Design review of the part shown in the three views and the two pictorial views. Dimensions are in mm from the part's minimum x, y and z. A direction names the side the tool comes from. Round coordinates to 2 decimals unless told otherwise and drop trailing zeros. Loops run counter-clockwise (first coordinate to the right, second up) from the corner with the lowest first, then second, coordinate; pieces in that order, holes last. Notation, with made-up numbers: (81, 63) -> (138, 63) arc R25 ccw to (138, 96) -> close; hole circle Ø6 at (57.25, 60.5). An arc over 180 degrees is marked (long way). Use CSV: the item, a comma, the result in double quotes. Start each with the question number.
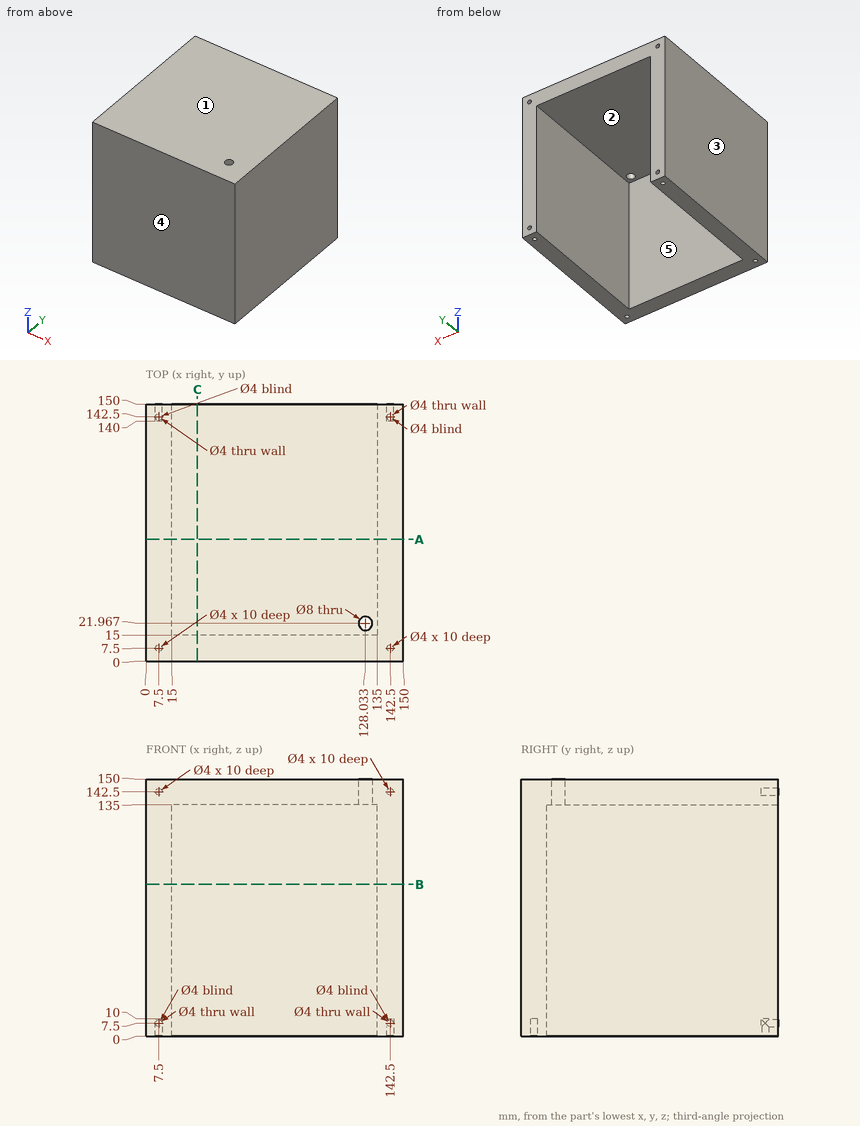
1. For the marked faces 1 and 2, list the 3-axis set-ups (+Z, -Z, +X, -X, +Y, -Y) from which the entire face can be reached by the end or side of a thin tool; tool diameter is ignored.
2. Take a section at C-C, the plane x = 30. Give the boundary of the cut face in (y, z).
3. Clearance check with flat-ended pins moving along their axes: P1, Ø4, axis at x = 78, z = 57.5, coming from the +Y side; P2, Ø8, axis at x = 92.5, y = 122.5, coming from the -Z side; P3, Ø2.5, axis at x = 7.5, z = 7.5, coming from the +Y side. State where each tip first meets the part, or that it passes through.
4. The part is to be moulded in two halves that separate along X. For the marked faces 3, 4 and 5, say which applies: pulls with the +X half, pulls with the -X half, needs draft (parallel to the pull), parting line crosses it, or undercut.
5. For line 1 along X through (y, z) = (142.5, 3.75); line 2 along X through (y, z) = (146.75, 142.5), list the stretches that pass through material, from the lowest coordinate up. Write a range as from..to.
6. Take a section at A-A, the plane y = 71. Give the boundary of the cut face in (x, z).
7. Take a section at B-B, the plane z = 88.5. Give the boundary of the cut face in (x, y), then the cut area to 3 significant figures.
Results:
1,face 1,"+Z, +X, -X, +Y, -Y"
1,face 2,"-Z, +Y"
2,outline,"(0, 0) -> (15, 0) -> (15, 135) -> (150, 135) -> (150, 150) -> (0, 150) -> close"
3,P1,"y = 15"
3,P2,"z = 135"
3,P3,"y = 140"
4,face 3,"pulls with the -X half"
4,face 4,"needs draft"
4,face 5,"undercut"
5,line 1,"0..5.5, 9.5..15, 135..140.5, 144.5..150"
5,line 2,"0..5.5, 9.5..140.5, 144.5..150"
6,outline,"(0, 0) -> (15, 0) -> (15, 135) -> (135, 135) -> (135, 0) -> (150, 0) -> (150, 150) -> (0, 150) -> close"
7,outline,"(0, 0) -> (150, 0) -> (150, 150) -> (135, 150) -> (135, 15) -> (15, 15) -> (15, 150) -> (0, 150) -> close"
7,area,"6,300 mm²"
